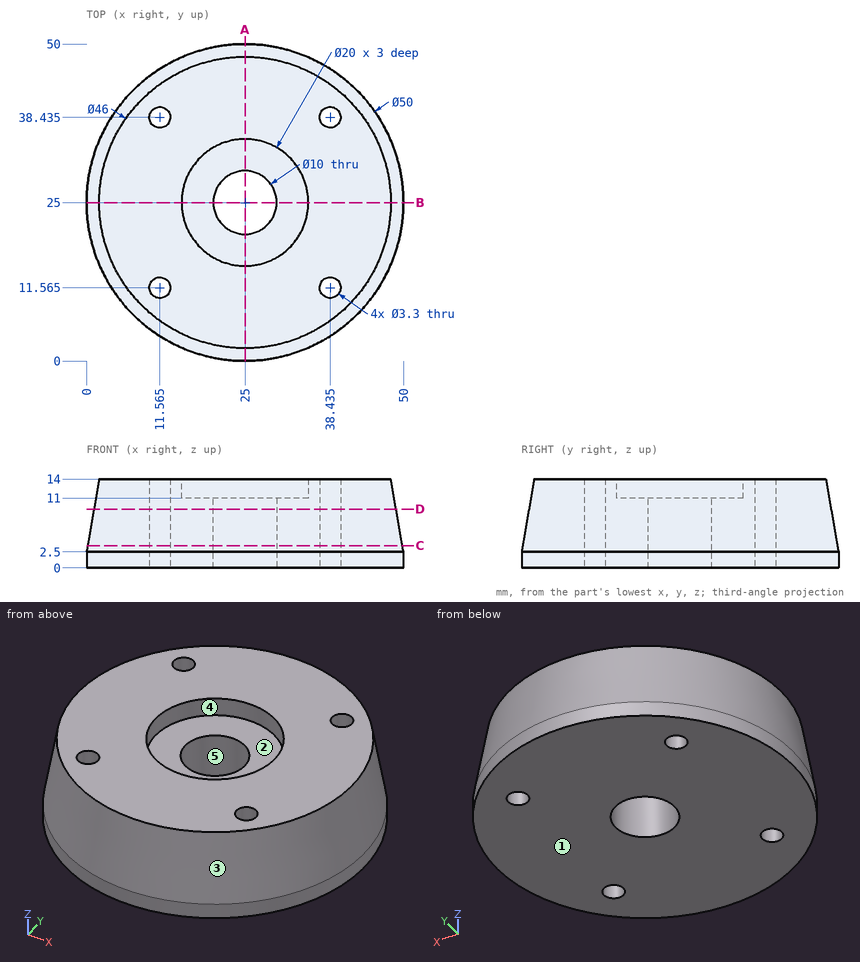
Answer from the drawing. Dimensions are ordinates in mm from the lowest x, y and z of the part. A direction names the side the tool comes from. Round coordinates to 2 decimals unless told otherwise and drop trailing zeros. Loops run counter-clockwise (first coordinate to the right, second up) from the corner with the lowest first, then second, coordinate; pieces in that order, holes last.
(1) Find the intervals of material crossed by L1, parallel to Z at x = 18.5, y = 21.5; L2, parallel to X at y = 37, z = 8.75; L3, parallel to Y at x = 29, z = 4.5, in increasing order.
Computed values:
L1: z = 0 to 11
L2: x = 4.32 to 10.75, 12.38 to 37.62, 39.25 to 45.68
L3: y = 0.67 to 22, 28 to 49.33
(2) The part is cut by section A-A, the plane x = 25. Give the vertices of the cut face in (y, z).
Computed values:
outline: (0, 0) - (20, 0) - (20, 11) - (15, 11) - (15, 14) - (2, 14) - (0, 2.5) - close; (30, 0) - (50, 0) - (50, 2.5) - (48, 14) - (35, 14) - (35, 11) - (30, 11) - close
(3) Each of these flat-tipped pins is pushed along its axis until it touches: P1, Ø2.5, axis at x = 38.44, y = 11.56, coming from the +Z side; P2, Ø5, axis at x = 40, z = 6, coming from the -Y side; P3, Ø1.5, axis at x = 39, z = 11.5, coming from the -Y side; P4, Ø4, axis at y = 22, z = 8, coming from the -X side. Where does it stop, or does it pass through?
Computed values:
P1: passes through
P2: stops at y = 3.97
P3: stops at y = 5.65
P4: stops at x = 0.74
(4) The mould has two halves that part along Y. Classify the marked faces 1, 2 and 3: pulls with the +Y half, pulls with the -Y half, needs draft (parallel to the pull), parting line crosses it, or undercut.
Computed values:
face 1: needs draft
face 2: undercut
face 3: parting line crosses it
(5) The part is cut by section D-D, the plane z = 9.25. Give the vertices of the cut face in (x, y) (3 decimals).
Computed values:
outline: circle Ø47.652 at (25, 25); hole circle Ø3.3 at (11.565, 11.565); hole circle Ø3.3 at (11.565, 38.435); hole circle Ø10 at (25, 25); hole circle Ø3.3 at (38.435, 11.565); hole circle Ø3.3 at (38.435, 38.435)
(6) For the marked faces 4 and 5, determine the directions among +Z, -Z, +X, -X, +Y, -Y from which every point of the face is accessible in a straight line to the end or side of a thin tool.
Computed values:
face 4: +Z
face 5: +Z, -Z
(7) The part is cut by section C-C, the plane z = 3.5. Give the vertices of the cut face in (x, y) (3 decimals).
Computed values:
outline: circle Ø49.652 at (25, 25); hole circle Ø3.3 at (11.565, 11.565); hole circle Ø3.3 at (11.565, 38.435); hole circle Ø10 at (25, 25); hole circle Ø3.3 at (38.435, 11.565); hole circle Ø3.3 at (38.435, 38.435)
